Design review of the part built by this model. Coordinates are the model's own, in mm. Face numbers are marked on the shaded views. A direction names the side the tool comes from. Round coordinates to 2 decimals unless told otherwise and drop trailing zeros. Order: outer loops, then holes, each group sorted by start corner. A loop starts at its lowest first (then second) coordinate and runs counter-clockwise, first axis right, second up.
from build123d import *

# Parameters (mm, degrees)
SKETCH_1_W          = 37.3
SKETCH_1_H          = 50.2
SKETCH_1_W_2        = 27.3
SKETCH_1_H_2        = 40.2
EXTRUDE_1_DEPTH     = 18
SKETCH_1_2_W        = 27.3
SKETCH_1_2_H        = 40.2
EXTRUDE_2_DEPTH     = 2
SKETCH_2_R          = 4.2
CUT_EXTRUDE_2_DEPTH = 37.080916008
SKETCH_3_W          = 3.5
SKETCH_3_H          = 3.5
CUT_EXTRUDE_3_DEPTH = 36.125951944
SKETCH_4_W          = 8.5
SKETCH_4_H          = 9.2
SKETCH_4_W_2        = 3.5
SKETCH_4_H_2        = 3.5
EXTRUDE_3_DEPTH     = 3
SKETCH_5_W          = 27.3
SKETCH_5_H          = 6.5
EXTRUDE_4_DEPTH     = 2
SKETCH_6_W          = 11.5
SKETCH_6_H          = 1.5
CUT_EXTRUDE_4_DEPTH = 10
FILLET_1_R          = 1
FILLET_2_R          = 3
SKETCH_7_R          = 1.4
CUT_EXTRUDE_5_DEPTH = 10
CUT_EXTRUDE_6_REACH = 38.081
SKETCH_8_W          = 13.3
SKETCH_8_H          = 4


with BuildPart() as part:
    # 스케치1 → 보스-돌출1 (new body)
    with BuildSketch(Plane.XY):
        Rectangle(SKETCH_1_W, SKETCH_1_H)
        Rectangle(SKETCH_1_W_2, SKETCH_1_H_2, mode=Mode.SUBTRACT)
    extrude(amount=EXTRUDE_1_DEPTH)

    # 스케치1<2> → 보스-돌출2 (add)
    with BuildSketch(Plane.XY):
        Rectangle(SKETCH_1_2_W, SKETCH_1_2_H)
    extrude(amount=EXTRUDE_2_DEPTH)

    # 스케치2 → 컷-돌출2 (cut, through all)
    with BuildSketch(Plane.XY):
        with Locations((0, 11.9)):
            Circle(SKETCH_2_R)
    extrude(amount=CUT_EXTRUDE_2_DEPTH, mode=Mode.SUBTRACT)

    # 스케치3 → 컷-돌출3 (cut, through all)
    with BuildSketch(Plane.XY.offset(2)):
        with Locations((-11.25, -9.85)):
            Rectangle(SKETCH_3_W, SKETCH_3_H)
    extrude(amount=-CUT_EXTRUDE_3_DEPTH, mode=Mode.SUBTRACT)

    # 스케치4 → 보스-돌출3 (add)
    with BuildSketch(Plane.XY.offset(2)):
        Polygon((-13.65, -20.1), (13.65, -20.1), (13.65, 20.1), (4.25, 20.1), (-4.25, 20.1), (-13.65, 20.1), align=None)
        with Locations((0, 12)):
            Rectangle(SKETCH_4_W, SKETCH_4_H, mode=Mode.SUBTRACT)
        with Locations((-11.25, -9.85)):
            Rectangle(SKETCH_4_W_2, SKETCH_4_H_2, mode=Mode.SUBTRACT)
    extrude(amount=EXTRUDE_3_DEPTH)

    # 스케치5 → 보스-돌출4 (add)
    with BuildSketch(Plane.XY.offset(5)):
        with Locations((0, -16.85)):
            Rectangle(SKETCH_5_W, SKETCH_5_H)
    extrude(amount=EXTRUDE_4_DEPTH)

    # 스케치6 → 컷-돌출4 (cut)
    with BuildSketch(Plane(origin=(0, 25.1, 0), x_dir=(1, 0, 0), z_dir=(0, 1, 0))):
        with Locations((-1.1, -7.75)):
            Rectangle(SKETCH_6_W, SKETCH_6_H)
    extrude(amount=-CUT_EXTRUDE_4_DEPTH, mode=Mode.SUBTRACT)

    # 필렛1
    fillet_1_edges = [part.edges().sort_by_distance(p)[0] for p in [
        (13.65, -20.1, 12.5),
        (13.65, 20.1, 11.5),
        (-13.65, 20.1, 11.5),
        (-13.65, -20.1, 12.5),
    ]]
    fillet(fillet_1_edges, radius=FILLET_1_R)

    # 필렛2
    fillet_2_edges = [part.edges().sort_by_distance(p)[0] for p in [
        (18.65, -25.1, 9),
        (-18.65, -25.1, 9),
        (-18.65, 25.1, 9),
        (18.65, 25.1, 9),
    ]]
    fillet(fillet_2_edges, radius=FILLET_2_R)

    # 스케치7 → 컷-돌출5 (cut)
    with BuildSketch(Plane.XY.offset(18)):
        with Locations((-15.65, 22.1)):
            Circle(SKETCH_7_R)
        with Locations((15.65, 22.1)):
            Circle(SKETCH_7_R)
        with Locations((-15.65, -22.1)):
            Circle(SKETCH_7_R)
        with Locations((15.65, -22.1)):
            Circle(SKETCH_7_R)
    extrude(amount=-CUT_EXTRUDE_5_DEPTH, mode=Mode.SUBTRACT)

    # 컷-돌출6: up to this face of the body (flat: up to its plane)
    cut_extrude_6_end = Plane(part.part.faces().sort_by_distance((-1.1, 22.6, 7))[0])
    # 스케치8 → 컷-돌출6 (cut, up to the picked face)
    with BuildSketch(Plane.XY.offset(18), mode=Mode.PRIVATE) as cut_extrude_6_sk1:
        with Locations((0, 20.1)):
            Rectangle(SKETCH_8_W, SKETCH_8_H)
    cut_extrude_6_tool1 = split(extrude(cut_extrude_6_sk1.sketch, amount=-CUT_EXTRUDE_6_REACH, mode=Mode.PRIVATE), bisect_by=cut_extrude_6_end, keep=Keep.BOTH, mode=Mode.PRIVATE)
    add(cut_extrude_6_tool1.solids().sort_by(Axis((0, 20.1, 18), (0, 0, -1)))[0], mode=Mode.SUBTRACT)


solid = part.part
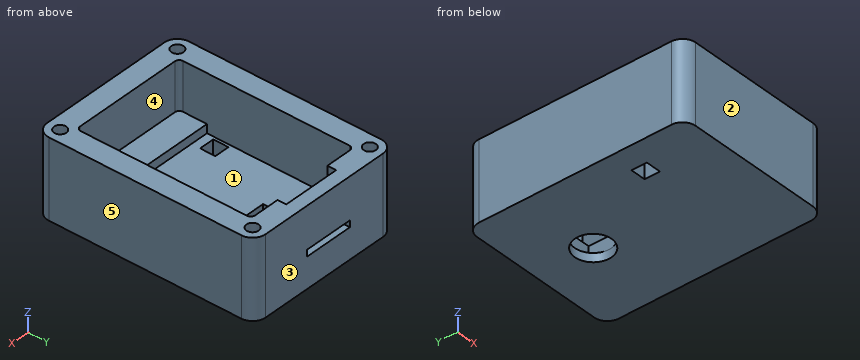
1) The part is to be moulded in two halves that separate along Y. For the marked faces 1, 2 and 3, say which applies: released by +Y, released by -Y, zero draft, split by the parting line, or undercut.
Results:
face 1: undercut
face 2: released by -Y
face 3: released by +Y
2) For the marked faces 4 and 5, list the 3-axis set-ups (+Z, -Z, +X, -X, +Y, -Y) from which the entire face can be reached by the end or side of a thin tool; tool diameter is ignored.
Results:
face 4: +Z
face 5: +Z, -Z, +X, +Y, -Y
3) Take a section at D-D on z = 4.25. Give the boundary of the cut face in (x, y).
Results:
outline: (-18.65, -22.1) arc R3 ccw to (-15.65, -25.1) - (15.65, -25.1) arc R3 ccw to (18.65, -22.1) - (18.65, 22.1) arc R3 ccw to (15.65, 25.1) - (-15.65, 25.1) arc R3 ccw to (-18.65, 22.1) - close; hole (-13, -11.6) - (-9.5, -11.6) - (-9.5, -8.1) - (-13, -8.1) - close; hole (-4.25, 7.4) - (4.25, 7.4) - (4.25, 16.6) - (-4.25, 16.6) - close
4) Take a section at B-B on y = 11.9. Give the boundary of the cut face in (x, z), plus the area to 3 significant figures.
Results:
outline: (-18.65, 0) - (-4.2, 0) - (-4.2, 2) - (-4.25, 2) - (-4.25, 5) - (-13.65, 5) - (-13.65, 18) - (-18.65, 18) - close; (4.2, 0) - (18.65, 0) - (18.65, 18) - (13.65, 18) - (13.65, 5) - (4.25, 5) - (4.25, 2) - (4.2, 2) - close
area: 274 mm2
5) Take a section at A-A on x = 0. Give the boundary of the cut face in (y, z), plus the area to 3 significant figures.
Results:
outline: (-25.1, 0) - (7.7, 0) - (7.7, 2) - (7.4, 2) - (7.4, 5) - (-13.6, 5) - (-13.6, 7) - (-20.1, 7) - (-20.1, 18) - (-25.1, 18) - close; (16.1, 0) - (25.1, 0) - (25.1, 7) - (20.1, 7) - (20.1, 5) - (16.6, 5) - (16.6, 2) - (16.1, 2) - close; (22.1, 8.5) - (25.1, 8.5) - (25.1, 18) - (22.1, 18) - close
area: 323 mm2
6) Clearance check with flat-ended pins moving along their axes: P1, Ø12, axis at x = -7, y = 9.5, coming from the +Z side; P2, Ø0.8, axis at y = 23, z = 8, coming from the +X side. State where each tip first meets the part, or that it passes through.
Results:
P1: stops at z = 5
P2: stops at x = 18.61
7) Take a section at C-C on z = 10.5. Give the boundary of the cut face in (x, y).
Results:
outline: (-18.65, -22.1) arc R3 ccw to (-15.65, -25.1) - (15.65, -25.1) arc R3 ccw to (18.65, -22.1) - (18.65, 22.1) arc R3 ccw to (15.65, 25.1) - (-15.65, 25.1) arc R3 ccw to (-18.65, 22.1) - close; hole circle Ø2.8 at (-15.65, -22.1); hole circle Ø2.8 at (-15.65, 22.1); hole (-13.65, -19.1) arc R1 ccw to (-12.65, -20.1) - (12.65, -20.1) arc R1 ccw to (13.65, -19.1) - (13.65, 19.1) arc R1 ccw to (12.65, 20.1) - (6.65, 20.1) - (6.65, 22.1) - (-6.65, 22.1) - (-6.65, 20.1) - (-12.65, 20.1) arc R1 ccw to (-13.65, 19.1) - close; hole circle Ø2.8 at (15.65, -22.1); hole circle Ø2.8 at (15.65, 22.1)
8) To check wall thickness, follow line 1 along Y through (x, z) = (15.65, 11.75); line 2 along X through (y, z) = (19, 9.5); line 3 along Y through (x, z) = (10, 10.25). State the ranges of each line that lie inside material, in increasing order.
Results:
line 1: y = -25.1 to -23.5, -20.7 to 20.7, 23.5 to 25.1
line 2: x = -18.65 to -13.65, 13.65 to 18.65
line 3: y = -25.1 to -20.1, 20.1 to 25.1
